Check sheet for the modelled part. Datum: model origin and axes. Units: mm. Face numbers are marked on the shaded views. A direction names the side the tool comes from. Give positions to 0.01 mm unless a question says otherwise; leave off trailing zeros. Order: outer loops, then holes, each group sorted by start corner. A loop starts at its lowest first (then second) coordinate and runs counter-clockwise, first axis right, second up. Notation, with made-up numbers: (-36, 50.5) -> (10, 50.5) arc R22 cw to (10, 67.5) -> close; hole circle Ø7 at (-9.75, -39). An arc over 180 degrees is marked (long way). Answer in a Markdown table with one row per item. Add a question column.
(1) Thickness scan on L1, parallel to X at y = -0.5, z = 130; L2, parallel to Z at x = -6.5, y = 0; L3, parallel to X at y = 10, z = 57. Record the ranges inside material, lowest first. Write a range as [from, to].
(2) Release check for a two-part mould opening along Z. For the marked faces 4, 5 and 6 record: released by +Z, released by -Z, zero draft, split by the parting line, or undercut.
(3) Cross-section at C-C (x = 18). Record the cut outline in (y, z), then the cut area to 3 significant figures.
(4) Cross-section at B-B (z = 130). Record the cut outline in (x, y).
(5) Cross-section at D-D (y = 34.5). Record the cut outline in (x, z).
(6) Set-up check for the marked faces 1, 2 and 3: record each of +Z, -Z, +X, -X, +Y, -Y from which the full face is reachable in a straight line by a thin tool's end or side.
(7) Cross-section at A-A (y = 0). Record the cut outline in (x, z).
(8) Go/stop test with flat-tipped pins: pin 1 (1 mm diameter, centred on y = -10, z = 146, fed in from -X); pin 2 (2 mm diameter, centred on y = 56.5, z = 139, fed in from +X); pin 3 (6 mm diameter, centred on y = -7.5, z = 66, fed in from +X). Record where each tip stops, or that it passes through.
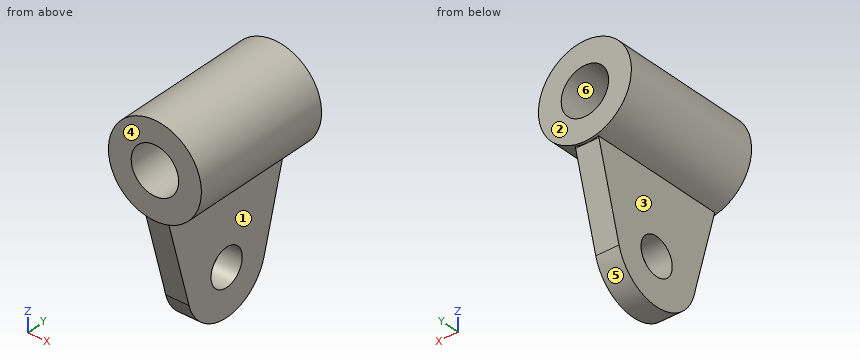
```python
from build123d import *

# Parameters (mm, degrees)
F0_R     = 20
F1_DEPTH = 12.5
F0_W     = 154
F0_H     = 24.5


# Not quite as in the source:
# - ends of sketch curves that miss each other by under 0.0002 mm in the source are joined


with BuildPart() as f1:
    # F0 (on Right) → F1 (new body, symmetric)
    with BuildSketch(Plane.YZ):
        with BuildLine():
            Line((73.9999998675, 80), (-73.9999998675, 80))
            Line((-73.9999998675, 80), (-48.191225, -13.326883))
            ThreePointArc((-48.191225, -13.326883), (0, -50), (48.1912252169, -13.32688306))
            Line((48.1912252169, -13.32688306), (73.9999998675, 80))
        make_face()
        Circle(F0_R, mode=Mode.SUBTRACT)
        Polygon((-77, 104.5), (-77, 90.848274), (-73.9999998675, 80), (73.9999998675, 80), (77, 90.848274), (77, 104.5), align=None)
    extrude(amount=F1_DEPTH, both=True)

    # F0 (on Right) → F2 (revolve)
    with BuildSketch(Plane.YZ):
        with Locations((0, 167.75)):
            Rectangle(F0_W, F0_H)
    revolve(axis=Axis((0, 0, 130), (0, 1, 0)))


solid = f1.part
```
Answer below:
| question | item | result |
|---|---|---|
| 1 | L1 | x = [-50, -25.5], [25.5, 50] |
| 1 | L2 | z = [-50, -20], [20, 105.34], [154.66, 179.58] |
| 1 | L3 | x = [-12.5, 12.5] |
| 2 | face 4 | zero draft |
| 2 | face 5 | released by -Z |
| 2 | face 6 | undercut |
| 3 | outline | (-77, 83.35) -> (77, 83.35) -> (77, 111.94) -> (-77, 111.94) -> close; (-77, 148.06) -> (77, 148.06) -> (77, 176.65) -> (-77, 176.65) -> close |
| 3 | area | 8,800 mm² |
| 4 | outline | (-50, -77) -> (-25.5, -77) -> (-25.5, 77) -> (-50, 77) -> close; (25.5, -77) -> (50, -77) -> (50, 77) -> (25.5, 77) -> close |
| 5 | outline | (-12.5, -36.19) -> (12.5, -36.19) -> (12.5, 81.59) arc R50 ccw (long way) to (-12.5, 81.59) -> close; hole circle Ø51 at (0, 130) |
| 6 | face 1 | -Z, +X, +Y, -Y |
| 6 | face 2 | +Z, -Z, +X, -X, +Y |
| 6 | face 3 | -Z, -X, +Y, -Y |
| 7 | outline | (-12.5, -50) -> (12.5, -50) -> (12.5, -20) -> (-12.5, -20) -> close; (-12.5, 20) -> (12.5, 20) -> (12.5, 81.59) arc R50 ccw (long way) to (-12.5, 81.59) -> close; hole circle Ø51 at (0, 130) |
| 8 | pin 1 | stops at x = -47.54 |
| 8 | pin 2 | stops at x = 49.36 |
| 8 | pin 3 | stops at x = 12.5 |
